```python
from build123d import *

# Parameters (mm, degrees)
SKETCH_FOR_MAIN_SHAPE_W = 88
SKETCH_FOR_MAIN_SHAPE_H = 91
MAIN_SHAPE_DEPTH        = 10
HOLLOW_T                = -1.8
FILLETS_R               = 1


with BuildPart() as part:
    # Sketch for main shape → Main shape (new body)
    with BuildSketch(Plane.XY):
        with Locations((44, 45.5)):
            Rectangle(SKETCH_FOR_MAIN_SHAPE_W, SKETCH_FOR_MAIN_SHAPE_H)
    extrude(amount=MAIN_SHAPE_DEPTH)

    # Hollow
    hollow_openings = [part.faces().sort_by_distance(p)[0] for p in [
        (44, 45.5, 10),
    ]]
    offset(amount=HOLLOW_T, openings=hollow_openings, kind=Kind.INTERSECTION)

    # Fillets
    fillets_edges = [part.edges().sort_by_distance(p)[0] for p in [
        (44, 91, 0),
        (88, 45.5, 0),
        (44, 0, 0),
        (0, 45.5, 0),
        (0, 91, 5),
        (88, 91, 5),
        (88, 0, 5),
        (0, 0, 5),
    ]]
    fillet(fillets_edges, radius=FILLETS_R)


solid = part.part
```
Work out the finished part from the listing and answer in its coordinate system (mm). A direction names the side the tool comes from. Round coordinates to 2 decimals unless told otherwise and drop trailing zeros. Write each loop counter-clockwise with the first axis right and the second up, starting at its lowest first coordinate (ties: lowest second). Pieces come first, ordered by that corner, then holes. Notation, with made-up numbers: (82, -6.5) - (127, -6.5) arc R13 cw to (127, 9.5) - close; hole circle Ø4 at (18, 88). An arc over 180 degrees is marked (long way). Return JSON: item names as keys, results as strings. Group by question number.
Q1. The part is cut by section C-C on y = 15.5. Write down the section's boundary in (x, z).
Q2. For faces 1 (the flat face through (1.8, 45, 6)), 2 (the flat face through (43, 0, 5)), determine the directions among +Z, -Z, +X, -X, +Y, -Y from which every point of the face is accessible in a straight line to the end or side of a thin tool.
Q3. The part is cut by section B-B on x = 40.5. Write down the section's boundary in (y, z).
Q4. This flat-tipped pin is pushed along its axis until it touches: pin 1 Ø3 at (x, y) = (31, 60) entering from +Z. Where does it stop, or does it pass through?
Q5. The mould has two halves that part along X. Classify faces 3 (the flat face through (43, 1.8, 6)), 4 (the flat face through (1, 66, 10)), 5 (the flat face through (88, 45, 5)), 6 (the flat face through (0, 45, 5)): released by +X, released by -X, zero draft, split by the parting line, or undercut.
Q6. Find the intervals of material crossed by L1, parallel to Y at x = 43, z = 4.25; L2, parallel to X at y = 79, z = 3.25; L3, parallel to Z at x = 16.5, y = 37.5, in increasing order.
Q7. The part is cut by section A-A on z = 5.5. Write down the section's boundary in (x, y).
Solved:
{
 "1": {"outline": "(0, 1) arc R1 ccw to (1, 0) - (87, 0) arc R1 ccw to (88, 1) - (88, 10) - (86.2, 10) - (86.2, 1.8) - (1.8, 1.8) - (1.8, 10) - (0, 10) - close"},
 "2": {"face 1": "+Z", "face 2": "+Z, -Z, +X, -X, -Y"},
 "3": {"outline": "(0, 1) arc R1 ccw to (1, 0) - (90, 0) arc R1 ccw to (91, 1) - (91, 10) - (89.2, 10) - (89.2, 1.8) - (1.8, 1.8) - (1.8, 10) - (0, 10) - close"},
 "4": {"pin 1": "z = 1.8"},
 "5": {"face 3": "undercut", "face 4": "zero draft", "face 5": "released by +X", "face 6": "released by -X"},
 "6": {"L1": "0 to 1.8, 89.2 to 91", "L2": "0 to 1.8, 86.2 to 88", "L3": "0 to 1.8"},
 "7": {"outline": "(0, 1) arc R1 ccw to (1, 0) - (87, 0) arc R1 ccw to (88, 1) - (88, 90) arc R1 ccw to (87, 91) - (1, 91) arc R1 ccw to (0, 90) - close; hole (1.8, 1.8) - (86.2, 1.8) - (86.2, 89.2) - (1.8, 89.2) - close"}
}
